Model file for the job. Use its own axes, mm. Face numbers are marked on the shaded views. Coordinates: 2 decimals unless noted, no trailing zeros. Write each loop counter-clockwise with the first axis right and the second up, starting at its lowest first coordinate (ties: lowest second). Pieces come first, ordered by that corner, then holes.
Q1. Pin check, flat tips, straight feed: P1, Ø4, axis at x = 4.5, y = 3, coming from the -Z side; P2, Ø10, axis at x = 8, z = -9.5, coming from the +Y side; P3, Ø1, axis at x = 11, z = -2, coming from the +Y side. Stop position of each tip, or through.
Q2. Drill centre lines: probe 1 along Z at (x, y) = (8, 0); probe 2 along X at (y, z) = (14.5, 3); probe 3 along Z at (x, y) = (2.75, 9). Where is each one in solid material? Low to high.
Q3. Band-saw the part on A-A, the plane x = 9. Write the cut outline in (y, z), plus the area to 3 significant figures.
Q4. Pull direction Y, two halves, no side cores. Call the marked faces 1, 2 and 3: released by +Y, released by -Y, zero draft, split by the parting line, or undercut.
Autodesk Inventor part; units mm, degrees
ref_plane "YZ Plane" through (0, 0, 0) normal (1, 0, 0) x (0, 1, 0)
ref_plane "XZ Plane" through (0, 0, 0) normal (0, 1, 0) x (-1, 0, 0)
ref_plane "XY Plane" through (0, 0, 0) normal (0, 0, 1) x (1, 0, 0)
sketch "Sketch1" plane through (0, 0, 0) normal (0, 0, 1) x (1, 0, 0)
  line L0 (0, 0) -> (19, 0)
  line L1 (0, 0) -> (0, 12.5) construction
  line L2 (0, 12.5) -> (0, 16.3)
  line L3 (0, 16.3) -> (2.85, 16.3)
  line L4 (2.85, 16.3) -> (2.85, 14.4)
  line L5 (2.85, 14.4) -> (19, 14.4)
  line L6 (0, 12.5) -> (19, 12.5)
  line L7 (19, 14.4) -> (19, 0) construction
  line L8 (19, 14.4) -> (22.8, 14.4) construction
  line L9 (22.8, 14.4) -> (22.8, 0) construction
  line L10 (22.8, 0) -> (19, 0) construction
  line L11 (20.9, 14.4) -> (20.9, 0) construction
  line L12 (19, -14.4) -> (19, 0) construction
  line L13 (19, -14.4) -> (22.8, -14.4) construction
  line L14 (22.8, -14.4) -> (22.8, 0) construction
  line L15 (20.9, -14.4) -> (20.9, 0) construction
  line L16 (20.9, 0) -> (19, 0) construction
  line L17 (19, 12.5) -> (19, 14.4)
  arc A0 (20.9, 0) -> (19, 12.5) centre (-21.1684, 0) ccw
  line L18 (19, 14.4) -> (20.3751, 14.4)
  line L19 (20.9, 0) -> (22.8, 0)
  arc A1 (22.8, 0) -> (20.3751, 14.4) centre (-21.1684, 0) ccw
  dimension "d0" = 2.85
  dimension "d2" = 1.9
  dimension "d3" = 1.9
  dimension "d4" = 25
  dimension "d5" = 19
  dimension "d6" = 3.8
revolve "Revolve1" add sketch "Sketch1" angle 360 about axis through (0, 0, 0) along (1, 0, 0) contours L2 L3 L4 L5 L17 L6
revolve "Revolve2" add sketch "Sketch1" angle 360 about axis through (20.9, 0, 0) along (-1, 0, 0) contours L17 L18 A1 L19 A0
equation "\"d0\" = 1.5 * s1"
equation "\"d2\" = s1"
equation "\"d3\" = s1"
equation "\"d4\" = d1"
equation "\"d5\" = t1"
equation "\"d6\" = 2 * s1"
equation "\"d1\" = 25"
equation "\"t1\" = 19"
equation "\"s1\" = 1.9"
properties part number "DIN 8063 Cap Type K 25" material "PVC, Unplasticized"
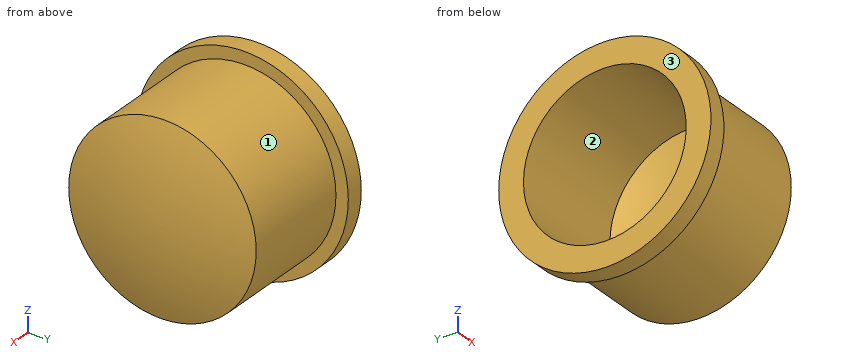
Answer sheet:
1. P1: stops at z = -16.19
1. P2: stops at y = 13.68
1. P3: stops at y = 14.32
2. probe 1: z = -14.4 to -12.5, 12.5 to 14.4
2. probe 2: x = 0 to 2.85
2. probe 3: z = -13.59 to -8.67, 8.67 to 13.59
3. outline: circle Ø28.8 at (0, 0); hole circle Ø25 at (0, 0)
3. area: 161 mm2
4. face 1: split by the parting line
4. face 2: undercut
4. face 3: zero draft
